Work out the finished part from the listing and answer in its coordinate system (mm). A direction names the side the tool comes from. Round coordinates to 2 decimals unless told otherwise and drop trailing zeros. Order: outer loops, then holes, each group sorted by start corner. A loop starts at its lowest first (then second) coordinate and runs counter-clockwise, first axis right, second up. Notation, with made-up numbers: (-12, 89.5) - (37, 89.5) arc R8 ccw to (37, 98.5) - close; hole circle Ø1 at (53.5, 85.25). An arc over 180 degrees is marked (long way). Answer in a Markdown table with one row per item.
from build123d import *

# Parameters (mm, degrees)
WHEEL_SUPPORT_RAILS_1_PROFILE_R       = 1.7
WHEEL_SUPPORT_RAILS_1_EXTRUSION_DEPTH = 3
WHEEL_SUPPORT_RAILS_2_EXTRUSION_DEPTH = 3
WHEEL_SUPPORT_RAILS_3_EXTRUSION_DEPTH = 0.1
WHEEL_SUPPORT_RAILS_4_EXTRUSION_DEPTH = 0.1
PIVOT_BACKING_5_EXTRUSION_DEPTH       = 59.3


with BuildPart() as part:
    # Wheel support rails 1 profile → Wheel support rails 1 extrusion (new body)
    with BuildSketch(Plane(origin=(0, -200, 0), x_dir=(1, 0, 0), z_dir=(0, 1, 0))):
        with BuildLine():
            Line((-19.3635199, 72.551817663), (-19.796031534, 72.551817663))
            Line((-19.796031534, 72.551817663), (-19.796031534, 77.344882879))
            Line((-19.796031534, 77.344882879), (-18.287181296, 77.344882879))
            ThreePointArc((-18.287181296, 77.344882879), (-19.831302101, 79.707937327), (-22.409182889, 80.858096458))
            Line((-22.409182889, 80.858096458), (-22.409182889, 77.466920099))
            ThreePointArc((-22.409182889, 77.466920099), (-21.643496924, 74.985063993), (-24.218406931, 74.644882879))
            Line((-24.218406931, 74.644882879), (-27.913875328, 74.644882879))
            ThreePointArc((-27.913875328, 74.644882879), (-27.347266001, 73.305528815), (-26.419206918, 72.185876289))
            ThreePointArc((-26.419206918, 72.185876289), (-35.919758288, 55.293042834), (-29.496951386, 37.007096044))
            ThreePointArc((-29.496951386, 37.007096044), (-29.716475974, 28.670321551), (-21.957552332, 31.727951993))
            ThreePointArc((-21.957552332, 31.727951993), (-2.577653733, 31.946649884), (10.047037269, 46.651937219))
            ThreePointArc((10.047037269, 46.651937219), (17.37665806, 50.630210597), (10.849210599, 55.820820355))
            ThreePointArc((10.849210599, 55.820820355), (5.348356993, 68.520951403), (-6.346539744, 75.922445127))
            Line((-6.346539744, 75.922445127), (-6.346539744, 73.320286475))
            ThreePointArc((-6.346539744, 73.320286475), (4.101805551, 66.093036958), (8.470715341, 54.163507116))
            ThreePointArc((8.470715341, 54.163507116), (7.414711079, 51.501768024), (7.992466121, 48.697093513))
            ThreePointArc((7.992466121, 48.697093513), (-3.634199387, 34.212419351), (-22.203580069, 34.616445929))
            ThreePointArc((-22.203580069, 34.616445929), (-23.98071161, 36.861841994), (-26.698508507, 37.763828705))
            ThreePointArc((-26.698508507, 37.763828705), (-33.429271543, 55.075153477), (-23.794683922, 70.954695591))
            ThreePointArc((-23.794683922, 70.954695591), (-21.379253869, 71.198784638), (-19.3635199, 72.551817663))
        make_face()
        with Locations(Location((12.395684569, 51.06598931, 0), (0, 0, 270))):
            Circle(WHEEL_SUPPORT_RAILS_1_PROFILE_R, mode=Mode.SUBTRACT)
        with Locations(Location((-26.848593792, 32.766081772, 0), (0, 0, 270))):
            Circle(WHEEL_SUPPORT_RAILS_1_PROFILE_R, mode=Mode.SUBTRACT)
    extrude(amount=WHEEL_SUPPORT_RAILS_1_EXTRUSION_DEPTH)

    # Wheel support rails 2 profile → Wheel support rails 2 extrusion (add)
    # profile 1 of 2: a face of its own
    with BuildSketch(Plane(origin=(0, -197, 0), x_dir=(1, 0, 0), z_dir=(0, 1, 0))):
        with BuildLine():
            Line((-19.3635199, 72.551817663), (-19.796031533, 72.551817663))
            Line((-19.796031533, 72.551817663), (-19.796031533, 75.86552534))
            Line((-19.796031533, 75.86552534), (-21.424639427, 73.044693722))
            Line((-21.424639427, 73.044693722), (-24.724639427, 73.044693722))
            Line((-24.724639427, 73.044693722), (-25.648509068, 74.644882879))
            Line((-25.648509068, 74.644882879), (-27.913875328, 74.644882879))
            ThreePointArc((-27.913875328, 74.644882879), (-27.347266001, 73.305528815), (-26.419206918, 72.185876289))
            ThreePointArc((-26.419206918, 72.185876289), (-35.919758288, 55.293042834), (-29.496951386, 37.007096044))
            ThreePointArc((-29.496951386, 37.007096044), (-29.716475974, 28.670321551), (-21.957552332, 31.727951993))
            ThreePointArc((-21.957552332, 31.727951993), (-2.577653733, 31.946649884), (10.047037269, 46.651937219))
            ThreePointArc((10.047037269, 46.651937219), (17.37665806, 50.630210597), (10.849210599, 55.820820355))
            ThreePointArc((10.849210599, 55.820820355), (5.348356993, 68.520951403), (-6.346539744, 75.922445127))
            Line((-6.346539744, 75.922445127), (-6.346539744, 73.320286475))
            ThreePointArc((-6.346539744, 73.320286475), (4.101805551, 66.093036958), (8.470715341, 54.163507116))
            ThreePointArc((8.470715341, 54.163507116), (7.414711079, 51.501768024), (7.992466121, 48.697093513))
            ThreePointArc((7.992466121, 48.697093513), (-3.634199387, 34.212419351), (-22.203580069, 34.616445929))
            ThreePointArc((-22.203580069, 34.616445929), (-23.98071161, 36.861841994), (-26.698508507, 37.763828705))
            ThreePointArc((-26.698508507, 37.763828705), (-33.429271543, 55.075153477), (-23.794683922, 70.954695591))
            ThreePointArc((-23.794683922, 70.954695591), (-21.379253869, 71.198784638), (-19.3635199, 72.551817663))
        make_face()
        Polygon((9.095684569, 51.06598931), (10.745684569, 53.923873143), (14.045684569, 53.923873143), (15.695684569, 51.06598931), (14.045684569, 48.208105478), (10.745684569, 48.208105478), align=None, mode=Mode.SUBTRACT)
        Polygon((-30.148593792, 32.766081772), (-28.498593792, 35.623965604), (-25.198593792, 35.623965604), (-23.548593792, 32.766081772), (-25.198593792, 29.908197939), (-28.498593792, 29.908197939), align=None, mode=Mode.SUBTRACT)
    # profile 2 of 2: a face of its own
    with BuildSketch(Plane(origin=(0, -197, 0), x_dir=(1, 0, 0), z_dir=(0, 1, 0))):
        with BuildLine():
            Line((-22.409182889, 78.760461387), (-21.424639427, 78.760461387))
            Line((-21.424639427, 78.760461387), (-19.796031533, 75.939629769))
            Line((-19.796031533, 75.939629769), (-19.796031533, 77.344882879))
            Line((-19.796031533, 77.344882879), (-18.287181296, 77.344882879))
            ThreePointArc((-18.287181296, 77.344882879), (-19.831302101, 79.707937327), (-22.409182889, 80.858096458))
            Line((-22.409182889, 80.858096458), (-22.409182889, 78.760461387))
        make_face()
    extrude(amount=WHEEL_SUPPORT_RAILS_2_EXTRUSION_DEPTH)

    # Wheel support rails 3 profile → Wheel support rails 3 extrusion (add)
    with BuildSketch(Plane(origin=(0, -194, 0), x_dir=(1, 0, 0), z_dir=(0, 1, 0))):
        with BuildLine():
            Line((9.095684569, 51.06598931), (10.745684569, 53.923873143))
            Line((10.745684569, 53.923873143), (10.981005967, 53.923873143))
            ThreePointArc((10.981005967, 53.923873143), (5.95177331, 67.785965934), (-6.346539744, 75.922445127))
            Line((-6.346539744, 75.922445127), (-6.346539744, 73.320286475))
            ThreePointArc((-6.346539744, 73.320286475), (-11.915808048, 32.253267736), (-19.796031533, 72.940106583))
            Line((-19.796031533, 72.940106583), (-19.796031533, 75.586589097))
            ThreePointArc((-19.796031533, 75.586589097), (-19.895657477, 75.553849531), (-19.99513633, 75.520665715))
            Line((-19.99513633, 75.520665715), (-21.424639427, 73.044693721))
            Line((-21.424639427, 73.044693721), (-24.724639427, 73.044693721))
            Line((-24.724639427, 73.044693721), (-24.842300126, 73.24848803))
            ThreePointArc((-24.842300126, 73.24848803), (-35.923839859, 55.245842318), (-28.057599985, 35.623965605))
            Line((-28.057599985, 35.623965605), (-25.198593791, 35.623965605))
            Line((-25.198593791, 35.623965605), (-23.548593792, 32.766081772))
            Line((-23.548593792, 32.766081772), (-23.666254491, 32.562287463))
            ThreePointArc((-23.666254491, 32.562287463), (-2.534736101, 31.966715397), (10.525187666, 48.590017317))
            Line((10.525187666, 48.590017317), (9.095684569, 51.06598931))
        make_face()
    extrude(amount=WHEEL_SUPPORT_RAILS_3_EXTRUSION_DEPTH)

    # Wheel support rails 4 profile → Wheel support rails 4 extrusion (add)
    with BuildSketch(Plane(origin=(0, -193.9, 0), x_dir=(1, 0, 0), z_dir=(0, 1, 0))):
        with BuildLine():
            Line((-6.346539744, 75.922445127), (-6.346539744, 73.320286475))
            ThreePointArc((-6.346539744, 73.320286475), (-11.915808048, 32.253267736), (-19.796031533, 72.940106583))
            Line((-19.796031533, 72.940106583), (-19.796031533, 75.586589097))
            ThreePointArc((-19.796031533, 75.586589097), (-20.77224205, 75.244243169), (-21.732439848, 74.859265381))
            ThreePointArc((-21.732439848, 74.859265381), (-22.356188381, 74.361854317), (-23.138165192, 74.203764887))
            ThreePointArc((-23.138165192, 74.203764887), (-35.919758287, 55.293042834), (-26.616158734, 34.450116791))
            ThreePointArc((-26.616158734, 34.450116791), (-25.873513849, 34.158640248), (-25.345615983, 33.560473178))
            ThreePointArc((-25.345615983, 33.560473178), (-2.577653732, 31.946649884), (10.821049933, 50.425266465))
            ThreePointArc((10.821049933, 50.425266465), (10.702153582, 51.214154072), (10.956232526, 51.97041057))
            ThreePointArc((10.956232526, 51.97041057), (6.540238452, 67.006043687), (-6.346539744, 75.922445127))
        make_face()
    extrude(amount=WHEEL_SUPPORT_RAILS_4_EXTRUSION_DEPTH)

    # Pivot backing 5 profile → Pivot backing 5 extrusion (add)
    with BuildSketch(Plane(origin=(0, -193.8, 0), x_dir=(1, 0, 0), z_dir=(0, 1, 0))):
        with BuildLine():
            Line((-6.346539744, 75.922445127), (-6.346539744, 73.320286475))
            ThreePointArc((-6.346539744, 73.320286475), (-11.915808048, 32.253267736), (-19.796031533, 72.940106583))
            Line((-19.796031533, 72.940106583), (-19.796031533, 75.586589097))
            ThreePointArc((-19.796031533, 75.586589097), (-11.922531942, 29.752206559), (-6.346539744, 75.922445127))
        make_face()
    extrude(amount=PIVOT_BACKING_5_EXTRUSION_DEPTH)


with BuildPart() as body_2:
    # Mirror1: mirrored copy
    add(part.part.mirror(Plane(origin=(0, 0, 0), x_dir=(0, 0, 1), z_dir=(0, -1, 0))))


solid = body_2.part
1) Find section D-D, the plane x = -10. Give the vertices of the cut face in (y, z), then the cut area to 3 significant figures.
Filled in:
| item | result |
|---|---|
| outline | (134.5, -32.4) - (200, -32.4) - (200, -29.88) - (134.5, -29.88) - close |
| area | 165 mm^2 |
2) Find section B-B, the plane z = -57. Give the vertices of the cut face in (x, y), then the cut area to 3 significant figures.
Filled in:
| item | result |
|---|---|
| outline | (-35.71, 134.5) - (-33.17, 134.5) - (-33.17, 200) - (-35.71, 200) - close; (8.15, 134.5) - (10.69, 134.5) - (10.69, 200) - (8.15, 200) - close |
| area | 332 mm^2 |
3) Find the intervals of material crossed by probe 1 along X at (y, z) = (180.5, -41.5); probe 2 along X at (y, z) = (186, -68); probe 3 along Z at (x, y) = (-29.5, 144), in increasing order. Write a range as from..to.
Filled in:
| item | result |
|---|---|
| probe 1 | x = -32.86..-29.92, 4.9..7.85 |
| probe 2 | x = -30.8..-27.45, 2.43..5.78 |
| probe 3 | z = -69.48..-65.59, -40.9..-37.01 |
4) Find section A-A, the plane x = -2. Give the vertices of the cut face in (y, z), then the cut area to 3 significant figures.
Filled in:
| item | result |
|---|---|
| outline | (134.5, -74.26) - (200, -74.26) - (200, -71.43) - (134.5, -71.43) - close; (134.5, -35.06) - (200, -35.06) - (200, -32.23) - (134.5, -32.23) - close |
| area | 372 mm^2 |
5) Each of these flat-tipped pins is pushed along its axis until it touches: pin 1 (6 mm diameter, centred on y = 183.5, z = -70.5, fed in from -X); pin 2 (2 mm diameter, centred on y = 183, z = -75, fed in from -X); pin 3 (0.9 mm diameter, centred on x = -23, y = 195, fed in from -Z); pin 4 (1 mm diameter, centred on x = -21.5, z = -38, fed in from +Y). Where does it stop, or does it pass through?
Filled in:
| item | result |
|---|---|
| pin 1 | stops at x = -31.19 |
| pin 2 | stops at x = -23.53 |
| pin 3 | stops at z = -73.04 |
| pin 4 | passes through |
6) The mould has two halves that part along Y. Classify faces 1 (the face through (7.42, 197.04, -51.54)), 2 (the face through (9.909, 195.472, -52.475)), 3 (the face through (-29, 194, -30)): released by +Y, released by -Y, zero draft, split by the parting line, or undercut.
Filled in:
| item | result |
|---|---|
| face 1 | zero draft |
| face 2 | undercut |
| face 3 | released by -Y |
7) Find section C-C, the plane y = 142.5. Give the vertices of the cut face in (x, z), then the cut area to 3 significant figures.
Filled in:
| item | result |
|---|---|
| outline | (-19.8, -75.59) - (-19.8, -72.94) arc R21 cw (long way) to (-6.35, -73.32) - (-6.35, -75.92) arc R23.5 ccw (long way) to start |
| area | 315 mm^2 |
8) Which of the six approach directions +Z, -Z, +X, -X, +Y, -Y give full straight-line access (tool end or side, diameter ignored) to faces 4 (the face through (-22, 193.9, -74)), 5 (the face through (-23, 195, -73.045)), 6 (the face through (14.882, 195.521, -49.657))?
Filled in:
| item | result |
|---|---|
| face 4 | -Z |
| face 5 | none |
| face 6 | -Y |
